Here's how the part is built. I have some questions about the finished solid (model axes, mm). A direction names the side the tool comes from. Coordinates: 2 decimals unless noted, no trailing zeros. Order: outer loops, then holes, each group sorted by start corner. A loop starts at its lowest first (then second) coordinate and runs counter-clockwise, first axis right, second up. Notation, with made-up numbers: M -23,47 L -5,47 A13 ccw -5,60 Z; hole C -3,-37.5 d11. An arc over 180 degrees is marked long. One line per question, with ' | ' between items. Start each with the question number.
```python
from build123d import *

# Parameters (mm, degrees)
F0_W     = 161.2
F0_H     = 10
F1_DEPTH = 1
F2_W     = 2
F2_H     = 10
F3_DEPTH = 10.2
F2_W_2   = 142.9
F4_DEPTH = 2
F6_DEPTH = 10


with BuildPart() as f1:
    # F0 (on Top) → F1 (new body)
    with BuildSketch(Plane.XY):
        Rectangle(F0_W, F0_H)
    extrude(amount=F1_DEPTH)

    # F2 (on face) → F3 (join)
    with BuildSketch(Plane.XY.offset(1)):
        with Locations((-79.6, 0)):
            Rectangle(F2_W, F2_H)
        with Locations((79.6, 0)):
            Rectangle(F2_W, F2_H)
    extrude(amount=F3_DEPTH)

    # F2 (on face) → F4 (join)
    with BuildSketch(Plane.XY.offset(1)):
        Rectangle(F2_W_2, F2_H)
    extrude(amount=F4_DEPTH)

    # F5 (on face) → F6 (join)
    with BuildSketch(Plane.XZ.offset(5)):
        Polygon((78.6, 11.2), (80.6, 11.2), (80.6, 17.199105), (76.6, 11.199105), (78.6, 11.199105), align=None)
        Polygon((-76.6, 11.2), (-80.6, 17.2), (-80.6, 11.2), (-78.6, 11.2), align=None)
    extrude(amount=-F6_DEPTH)


solid = f1.part
```
1. Imagine slicing it at A-A (z = 15.5). List the corners of the cut face in (x, y) for me.
2. Imagine slicing it at C-C (x = 70). List the corners of the cut face in (y, z) for me.
3. Which directions (+Z, -Z, +X, -X, +Y, -Y) give clear straight access to the entire face, cutting with the end or side of a thin tool? Please do faces 1 (the face through (-78.6, -0.1, 14.2)), 2 (the face through (78.6, 0, 6)), 3 (the face through (-1, 0, 0)).
4. Imagine slicing it at B-B (y = -0.5). List the corners of the cut face in (x, z) for me.
5. I need wall thicknesses on line 1 (X direction, y = -2.5, z = 1.75); line 2 (X direction, y = -1.75, z = 3.5); line 3 (Z direction, x = -8.5, y = 4). Which ranges of each line are inside material? Lowest first, please.
6. Will these pins go through, and if not, where does the flat tip stop? pin 1 (5 mm diameter, centred on x = -30.5, y = -2, fed in from +Z); pin 2 (5.5 mm diameter, centred on x = 75, y = 1, fed in from +Z); pin 3 (2 mm diameter, centred on x = -76, y = -2, fed in from +Z); pin 4 (1 mm diameter, centred on x = 56.5, z = 5, fed in from +Y).
7. We'd pull the mould along X, two halves only. Please class faces 4 (the face through (80.6, 0, 8)), 5 (the face through (-80.6, 0, 8)), 6 (the face through (-78.6, 0, 6)), 7 (the face through (-1, 0, 3)): released by +X, released by -X, zero draft, split by the parting line, or undercut.
Entries:
1) outline: M -80.6,-5 L -79.47,-5 L -79.47,5 L -80.6,5 Z; M 79.47,-5 L 80.6,-5 L 80.6,5 L 79.47,5 Z
2) outline: M -5,0 L 5,0 L 5,3 L -5,3 Z
3) face 1: +Z, +Y, -Y | face 2: +Y, -Y | face 3: -Z, +X, -X, +Y, -Y
4) outline: M -80.6,0 L 80.6,0 L 80.6,17.2 L 76.6,11.2 L 78.6,11.2 L 78.6,1 L 71.45,1 L 71.45,3 L -71.45,3 L -71.45,1 L -78.6,1 L -78.6,11.2 L -76.6,11.2 L -80.6,17.2 Z
5) line 1: -80.6 to -78.6, -71.45 to 71.45, 78.6 to 80.6 | line 2: -80.6 to -78.6, 78.6 to 80.6 | line 3: 0 to 3
6) pin 1: z = 3 | pin 2: z = 12.92 | pin 3: z = 11.8 | pin 4: through
7) face 4: released by +X | face 5: released by -X | face 6: undercut | face 7: undercut
